from build123d import *

# Parameters (mm, degrees)
F0_W     = 25.4
F0_H     = 22.86
F1_DEPTH = 25.4
F2_T     = -2.54
F4_DEPTH = 2.54


with BuildPart() as f1:
    # F0 (on Front) → F1 (new body)
    with BuildSketch(Plane.XZ):
        Rectangle(F0_W, F0_H)
    extrude(amount=F1_DEPTH)

    # F2
    f2_openings = [f1.faces().sort_by_distance(p)[0] for p in [
        (0, -12.7, 11.43),
    ]]
    offset(amount=F2_T, openings=f2_openings)

    # F3 (on face) → F4 (join)
    with BuildSketch(Plane.XY.offset(11.43)):
        Polygon((12.7, 0), (-12.7, 0), (-12.7, -25.4), (-10.16, -25.4), (-10.16, -2.54), (10.16, -2.54), (10.16, -25.4), (12.7, -25.4), align=None)
    extrude(amount=F4_DEPTH)


solid = f1.part
Work out the finished part from the listing and answer in its coordinate system (mm). A direction names the side the tool comes from. Round coordinates to 2 decimals unless told otherwise and drop trailing zeros. Loops run counter-clockwise (first coordinate to the right, second up) from the corner with the lowest first, then second, coordinate; pieces in that order, holes last. Notation, with made-up numbers: (48, 61) -> (86, 61) arc R31 cw to (86, 93) -> close; hole circle Ø1 at (8, 70.25). An arc over 180 degrees is marked (long way). Use one line per item in the form item = value.
(1) A tool of negligible diameter and unlimited length cuts with its end or side. For faces 4 (the flat face through (0, -24, 11.43)), 5 (the flat face through (0, -13, -8.89)), 6 (the flat face through (-1, -2, 13.97)), from which of +Z, -Z, +X, -X, +Y, -Y can it reach the whole face along a straight path? Write none if from no direction.
Answer list:
face_4 = +Z, -Y
face_5 = +Z
face_6 = +Z, +X, -X, +Y, -Y
(2) For a pull along Y with two mould halves and no side action, classify faces 1 (the flat face through (0, -2.54, 2)), 2 (the flat face through (0, -25.4, 1)), 3 (the flat face through (0, -13, -11.43)) as released by +Y, released by -Y, zero draft, split by the parting line, or undercut.
Answer list:
face_1 = undercut
face_2 = released by -Y
face_3 = zero draft
(3) Find section B-B on y = -23.5. Give the vertices of the cut face in (x, z), then the cut area to 3 significant figures.
Answer list:
outline = (-12.7, -11.43) -> (12.7, -11.43) -> (12.7, 13.97) -> (10.16, 13.97) -> (10.16, 11.43) -> (-10.16, 11.43) -> (-10.16, 13.97) -> (-12.7, 13.97) -> close
area = 594 mm2
(4) Flat-ended cylindrical pins translate along their axes: P1, Ø3, axis at x = 2.5, y = -24.5, coming from the +Z side; P2, Ø5, axis at x = 0.5, y = -8.5, coming from the +Z side. Find the tip coordinate at first contact, or state that the pin passes through.
Answer list:
P1 = 11.43
P2 = -8.89
(5) Straight lines are drawn through the part: line 1 (X direction, y = -20, z = -1.75); line 2 (Y direction, x = 10, z = 6); line 3 (Y direction, x = -1.25, z = 11.75). For each, find the intervals that lie inside material, in ascending order.
Answer list:
line_1 = -12.7 to -10.16, 10.16 to 12.7
line_2 = -25.4 to -22.86, -2.54 to 0
line_3 = -2.54 to 0
(6) Find section C-C on x = -8.5. Give the vertices of the cut face in (y, z), then the cut area to 3 significant figures.
Answer list:
outline = (-25.4, -11.43) -> (0, -11.43) -> (0, 13.97) -> (-2.54, 13.97) -> (-2.54, -8.89) -> (-22.86, -8.89) -> (-22.86, 11.43) -> (-25.4, 11.43) -> close
area = 174 mm2
(7) Find section A-A on z = 10. Give the vertices of the cut face in (x, y), then the cut area to 3 significant figures.
Answer list:
outline = (-12.7, -25.4) -> (12.7, -25.4) -> (12.7, 0) -> (-12.7, 0) -> close; hole (-10.16, -22.86) -> (10.16, -22.86) -> (10.16, -2.54) -> (-10.16, -2.54) -> close
area = 232 mm2
